Could you check a few things on this model? Use its own coordinates, in mm. Give positions to 0.01 mm unless a question says otherwise; leave off trailing zeros. Order: outer loops, then holes, each group sorted by start corner. A loop starts at its lowest first (then second) coordinate and runs counter-clockwise, first axis right, second up. Notation, with made-up numbers: (-3.75, 49) -> (16.25, 49) arc R27 ccw to (16.25, 78) -> close; hole circle Ø1 at (41, 14). An arc over 180 degrees is marked (long way). Answer as CSV lines item,"result". Start each with the question number.
(1) Will these pins go through, and if not, where does the flat tip stop? pin 1 Ø1 at (y, z) = (1.5, -195) entering from +X; pin 2 Ø1.8 at (x, y) = (512.5, 2) entering from -Z.
(2) I need wall thicknesses on L1, parallel to Z at x = 103.5, y = 2.85; L2, parallel to Z at x = 462, y = 2.65; L3, parallel to X at y = 1, z = -204. Which ranges of each line are inside material? Lowest first, please.
(3) I want a section at B-B (z = -180.5). Please give me the cut outline in (x, y).
(4) I want a section at A-A (y = 2.1). Please give me the cut outline in (x, z).
(5) I want a section at C-C (x = 491). Please give me the cut outline in (y, z), plus the area to 3 significant figures.
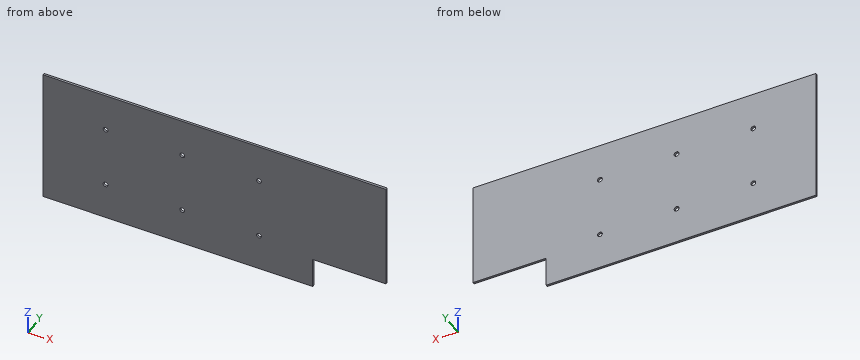
```python
from build123d import *

# Parameters (mm, degrees)
BOSS_EXTRUDE1_DEPTH     = 3.5
CUT_EXTRUDE1_DEPTH      = 602.385693628
CUT_EXTRUDE1_DEPTH_BACK = 602.385693628
SKETCH2_R               = 4


with BuildPart() as part:
    # Sketch1 → Boss-Extrude1 (new body)
    with BuildSketch(Plane(origin=(0, 0, 0), x_dir=(1, 0, 0), z_dir=(0, 1, 0))):
        Polygon((0, 0), (0, 222.25), (439.5, 222.25), (439.5, 172.8), (558.8, 172.8), (558.8, 0), align=None)
    extrude(amount=BOSS_EXTRUDE1_DEPTH)

    # Sketch2 → Cut-Extrude1 (cut, two sides: drawn at the far end of the back side and taken through both)
    with BuildSketch(Plane(origin=(0, 3.5, 0), x_dir=(1, 0, 0), z_dir=(0, 1, 0)).offset(-CUT_EXTRUDE1_DEPTH_BACK)):
        with Locations(Location((101.97168799, 162.2158083, 0), (0, 0, 270))):
            Circle(SKETCH2_R)
        with Locations(Location((226.97168799, 162.2158083, 0), (0, 0, 270))):
            Circle(SKETCH2_R)
        with Locations(Location((351.97168799, 162.2158083, 0), (0, 0, 270))):
            Circle(SKETCH2_R)
        with Locations(Location((351.97168799, 62.2158083, 0), (0, 0, 270))):
            Circle(SKETCH2_R)
        with Locations(Location((226.97168799, 62.2158083, 0), (0, 0, 270))):
            Circle(SKETCH2_R)
        with Locations(Location((101.97168799, 62.2158083, 0), (0, 0, 270))):
            Circle(SKETCH2_R)
    extrude(amount=CUT_EXTRUDE1_DEPTH + CUT_EXTRUDE1_DEPTH_BACK, mode=Mode.SUBTRACT)


solid = part.part
```
Final values:
1,pin 1,"x = 439.5"
1,pin 2,"z = -172.8"
2,L1,"-222.25 to -165.91, -158.52 to -65.91, -58.52 to 0"
2,L2,"-172.8 to 0"
2,L3,"0 to 439.5"
3,outline,"(0, 0) -> (439.5, 0) -> (439.5, 3.5) -> (0, 3.5) -> close"
4,outline,"(0, -222.25) -> (439.5, -222.25) -> (439.5, -172.8) -> (558.8, -172.8) -> (558.8, 0) -> (0, 0) -> close; hole circle Ø8 at (101.97, -162.22); hole circle Ø8 at (101.97, -62.22); hole circle Ø8 at (226.97, -162.22); hole circle Ø8 at (226.97, -62.22); hole circle Ø8 at (351.97, -162.22); hole circle Ø8 at (351.97, -62.22)"
5,outline,"(0, -172.8) -> (3.5, -172.8) -> (3.5, 0) -> (0, 0) -> close"
5,area,"605 mm²"
